from build123d import *

# Parameters (mm, degrees)
BOSS_EXTRUDE1_DEPTH = 1
SKETCH2_W           = 50
SKETCH2_H           = 11.4
BOSS_EXTRUDE2_DEPTH = 4.4
SKETCH3_R           = 2.25
CUT_EXTRUDE1_DEPTH  = 4.4
SKETCH4_W           = 50
SKETCH4_H           = 5.5
BOSS_EXTRUDE3_DEPTH = 6.4
SKETCH5_W           = 50
SKETCH5_H           = 4.5
BOSS_EXTRUDE4_DEPTH = 2
SKETCH6_W           = 50
SKETCH6_H           = 5.5
BOSS_EXTRUDE5_DEPTH = 2


with BuildPart() as part:
    # Sketch1 → Boss-Extrude1 (new body)
    with BuildSketch(Plane(origin=(0, 0, 0), x_dir=(0, 1, 0), z_dir=(0, 0, 1))):
        Polygon((-4, 25), (-4, 1), (19, 1), (19, 25), (25, 25), (25, -25), (-25, -25), (-25, 25), align=None)
    extrude(amount=BOSS_EXTRUDE1_DEPTH)

    # Sketch2 → Boss-Extrude2 (add)
    with BuildSketch(Plane.YZ.offset(25)):
        with Locations((0, -4.7)):
            Rectangle(SKETCH2_W, SKETCH2_H)
    extrude(amount=BOSS_EXTRUDE2_DEPTH)

    # Sketch3 → Cut-Extrude1 (cut)
    with BuildSketch(Plane.YZ.offset(29.4)):
        with Locations(Location((-20, -3.787139035, 0), (0, 0, 270))):
            Circle(SKETCH3_R)
        with Locations(Location((20, -3.787139035, 0), (0, 0, 270))):
            Circle(SKETCH3_R)
    extrude(amount=-CUT_EXTRUDE1_DEPTH, mode=Mode.SUBTRACT)

    # Sketch4 → Boss-Extrude3 (add)
    with BuildSketch(Plane(origin=(0, 0, 0), x_dir=(1, 0, 0), z_dir=(0, 0, -1))):
        with Locations((0, -22.25)):
            Rectangle(SKETCH4_W, SKETCH4_H)
        with Locations((0, 22.25)):
            Rectangle(SKETCH4_W, SKETCH4_H)
    extrude(amount=BOSS_EXTRUDE3_DEPTH)

    # Sketch5 → Boss-Extrude4 (add)
    with BuildSketch(Plane(origin=(0, 0, -6.4), x_dir=(1, 0, 0), z_dir=(0, 0, -1))):
        with Locations((0, 22.75)):
            Rectangle(SKETCH5_W, SKETCH5_H)
        with Locations((0, -22.75)):
            Rectangle(SKETCH5_W, SKETCH5_H)
    extrude(amount=BOSS_EXTRUDE4_DEPTH)

    # Sketch6 → Boss-Extrude5 (add)
    with BuildSketch(Plane(origin=(0, 0, -8.4), x_dir=(1, 0, 0), z_dir=(0, 0, -1))):
        with Locations((0, 22.25)):
            Rectangle(SKETCH6_W, SKETCH6_H)
        with Locations((0, -22.25)):
            Rectangle(SKETCH6_W, SKETCH6_H)
    extrude(amount=BOSS_EXTRUDE5_DEPTH)


solid = part.part
Verification items for the finished model (mm, model axes). A direction names the side the tool comes from. Coordinates: 2 decimals unless noted, no trailing zeros. Order: outer loops, then holes, each group sorted by start corner. A loop starts at its lowest first (then second) coordinate and runs counter-clockwise, first axis right, second up. Notation, with made-up numbers: (35.5, -6) -> (83.5, -6) arc R12 cw to (83.5, 3) -> close; hole circle Ø4 at (-18.5, 56.25). An arc over 180 degrees is marked (long way). Use CSV: the item, a comma, the result in double quotes. Start each with the question number.
Q1. Depth check by flat-ended pin: P1, Ø3, axis at x = 12, y = -11.5, coming from the -Z side. Enter the tip coordinate at first touch or a pass-through.
Q2. Section check D-D, the plane y = 4.5. Record the cut outline in (x, z).
Q3. Section check A-A, the plane x = -3. Record the cut outline in (y, z), and give its area (3 significant figures).
Q4. Section check C-C, the plane x = 24. Record the cut outline in (y, z), and give its area (3 significant figures).
Q5. Thickness scan on line 1 along Z through (x, y) = (26.05, 20); line 2 along Y through (x, z) = (23, -6.75); line 3 along Y through (x, z) = (-17, -0.75). Record the ranges inside material, lowest first.
Q6. Tool access check on faces 4 (the flat face through (0, -19.5, -9)), 5 (the flat face through (25, -21, -4)), 6 (the flat face through (0, -20.5, -7)). Record the directions out of +Z, -Z, +X, -X, +Y, -Y that give a thin tool (end or side, any length) a straight path to the whole face; none if there is none.
Q7. Section check B-B, the plane z = -5.25. Record the cut outline in (x, y), and give its area (3 significant figures).
Q8. Draft check along Y on faces 1 (the flat face through (29.4, 0, -5)), 2 (the cylindrical face through (27.231, -22.196, -3.299)), 3 (the flat face through (2, 25, -5)). Enter one of: +Y half, -Y half, draft (parallel to the pull), parting line (faces both ways), or undercut.
Returned:
1,P1,"stops at z = 0"
2,outline,"(-1, 0) -> (25, 0) -> (25, -10.4) -> (29.4, -10.4) -> (29.4, 1) -> (-1, 1) -> close"
3,outline,"(-25, -10.4) -> (-19.5, -10.4) -> (-19.5, -8.4) -> (-20.5, -8.4) -> (-20.5, -6.4) -> (-19.5, -6.4) -> (-19.5, 0) -> (-4, 0) -> (-4, 1) -> (-25, 1) -> close; (19, 0) -> (19.5, 0) -> (19.5, -6.4) -> (20.5, -6.4) -> (20.5, -8.4) -> (19.5, -8.4) -> (19.5, -10.4) -> (25, -10.4) -> (25, 1) -> (19, 1) -> close"
3,area,"137 mm^2"
4,outline,"(-25, -10.4) -> (-19.5, -10.4) -> (-19.5, -8.4) -> (-20.5, -8.4) -> (-20.5, -6.4) -> (-19.5, -6.4) -> (-19.5, 0) -> (19.5, 0) -> (19.5, -6.4) -> (20.5, -6.4) -> (20.5, -8.4) -> (19.5, -8.4) -> (19.5, -10.4) -> (25, -10.4) -> (25, 1) -> (-25, 1) -> close"
4,area,"160 mm^2"
5,line 1,"z = -10.4 to -6.04, -1.54 to 1"
5,line 2,"y = -25 to -20.5, 20.5 to 25"
5,line 3,"y = -25 to -19.5, 19.5 to 25"
6,face 4,"-Z, -X"
6,face 5,"+X"
6,face 6,"-X"
7,outline,"(-25, -25) -> (29.4, -25) -> (29.4, -21.71) -> (25, -21.71) -> (25, -19.5) -> (-25, -19.5) -> close; (-25, 19.5) -> (25, 19.5) -> (25, 21.71) -> (29.4, 21.71) -> (29.4, 25) -> (-25, 25) -> close; (25, -18.29) -> (29.4, -18.29) -> (29.4, 18.29) -> (25, 18.29) -> close"
7,area,"740 mm^2"
8,face 1,"draft"
8,face 2,"undercut"
8,face 3,"+Y half"
